```python
from build123d import *

# Parameters (mm, degrees)
EXTRUDE_1_DEPTH     = 18
SKETCH_3_W          = 20
SKETCH_3_H          = 30
EXTRUDE_2_DEPTH     = 2
SKETCH_4_W          = 4.85
SKETCH_4_H          = 30
EXTRUDE_3_DEPTH     = 6.5
EXTRUDE_START       = -20
SKETCH_5_W          = 3
SKETCH_5_H          = 12
EXTRUDE_4_DEPTH     = 20
SKETCH_2_R          = 1.25
CUT_EXTRUDE_1_DEPTH = 18


with BuildPart() as part:
    # 스케치1 → 보스-돌출1 (new body)
    with BuildSketch(Plane.XY):
        Polygon((-15, 12), (-15, 0), (15, 0), (15, 12), (11, 12), (11, 5), (-11, 5), (-11, 12), align=None)
    extrude(amount=EXTRUDE_1_DEPTH)

    # 스케치3 → 보스-돌출2 (add)
    with BuildSketch(Plane(origin=(0, 0, 0), x_dir=(-1, 0, 0), z_dir=(0, 0, -1))):
        with Locations((5, 15)):
            Rectangle(SKETCH_3_W, SKETCH_3_H)
    extrude(amount=EXTRUDE_2_DEPTH)

    # 스케치4 → 보스-돌출3 (add)
    with BuildSketch(Plane(origin=(0, 0, -2), x_dir=(-1, 0, 0), z_dir=(0, 0, -1))):
        with Locations((5, 15)):
            Rectangle(SKETCH_4_W, SKETCH_4_H)
    extrude(amount=EXTRUDE_3_DEPTH)

    # 스케치5 → 보스-돌출4 (add)
    with BuildSketch(Plane.XY.offset(18).offset(EXTRUDE_START)):
        with Locations((-16.5, -1)):
            Rectangle(SKETCH_5_W, SKETCH_5_H)
        with Locations((6.5, -1)):
            Rectangle(SKETCH_5_W, SKETCH_5_H)
    extrude(amount=EXTRUDE_4_DEPTH)

    # 스케치2 → 컷-돌출1 (cut)
    with BuildSketch(Plane(origin=(0, 5, 0), x_dir=(1, 0, 0), z_dir=(0, 1, 0))):
        with Locations((-4.8, -11.5)):
            Circle(SKETCH_2_R)
        with Locations((4.8, -11.5)):
            Circle(SKETCH_2_R)
    extrude(amount=-CUT_EXTRUDE_1_DEPTH, mode=Mode.SUBTRACT)


solid = part.part
```
Check sheet for the modelled part. Datum: model origin and axes. Units: mm. A direction names the side the tool comes from. Round coordinates to 2 decimals unless told otherwise and drop trailing zeros. Loops run counter-clockwise (first coordinate to the right, second up) from the corner with the lowest first, then second, coordinate; pieces in that order, holes last. Notation, with made-up numbers: (43, -14) - (90, -14) arc R19 ccw to (90, 0) - close; hole circle Ø11 at (6, -29.5). An arc over 180 degrees is marked (long way). Write item = value, one per line. Start each with the question number.
Q1. Section check A-A (z = 11.5). Record the boundary of the cut face in (x, y), plus the area to 3 significant figures.
Q2. Section check B-B (x = -4.8). Record the boundary of the cut face in (y, z), plus the area to 4 significant figures.
Q3. Thickness scan on L1, parallel to X at y = -1, z = -1.5; L2, parallel to X at y = 0.5, z = 11.5; L3, parallel to X at y = 10.5, z = 14. Record the ranges inside material, lowest first.
Q4. Section check D-D (x = 0.5). Record the boundary of the cut face in (y, z).
Q5. Release check for a two-part mould opening along X. For faces 4 (the face through (5.955, 0.417, 11.979)), 5 (the face through (-18, -1, 8)), 6 (the face through (5, 17, -1)) record: pulls with the +X half, pulls with the -X half, needs draft (parallel to the pull), parting line crosses it, or undercut.
Q6. Section check C-C (y = -5). Record the boundary of the cut face in (x, z), plus the area to 3 significant figures.
Q7. Access from +Z, -Z, +X, -X, +Y, -Y to the whole of each face (thin tool, end or side, straight path). Record for faces 1 (the face through (-11, 8, 9)), 2 (the face through (12, 5, 0)), 3 (the face through (11, 9, 9)).
Q8. Depth check by flat-ended pin: P1, Ø3.5, axis at x = -16.5, z = 8, coming from the +Y side; P2, Ø1, axis at x = 5, y = -2.5, coming from the -Z side; P3, Ø0.6, axis at y = 17, z = -0.5, coming from the +X side. Enter the tip coordinate at first touch or a pass-through.
Derived:
q1.outline = (-18, -7) - (-15, -7) - (-15, 0) - (-6.05, 0) - (-6.05, 5) - (-11, 5) - (-11, 12) - (-15, 12) - (-15, 5) - (-18, 5) - close; (-3.55, 0) - (3.55, 0) - (3.55, 5) - (-3.55, 5) - close; (6.05, -7) - (8, -7) - (8, 0) - (15, 0) - (15, 12) - (11, 12) - (11, 5) - (6.05, 5) - close
q1.area = 231 mm^2
q2.outline = (0, -8.5) - (30, -8.5) - (30, 0) - (5, 0) - (5, 10.25) - (0, 10.25) - close; (0, 12.75) - (5, 12.75) - (5, 18) - (0, 18) - close
q2.area = 332.5 mm^2
q3.L1 = -18 to -15, 5 to 8
q3.L2 = -18 to -6.05, -3.55 to 3.55, 6.05 to 15
q3.L3 = -15 to -11, 11 to 15
q4.outline = (0, -2) - (30, -2) - (30, 0) - (5, 0) - (5, 18) - (0, 18) - close
q5.face_4 = undercut
q5.face_5 = pulls with the -X half
q5.face_6 = pulls with the +X half
q6.outline = (-18, -2) - (-15, -2) - (-15, 18) - (-18, 18) - close; (5, -2) - (8, -2) - (8, 18) - (5, 18) - (5, 12.73) arc R1.25 cw to (5, 10.27) - close
q6.area = 118 mm^2
q7.face_1 = +Z, +Y
q7.face_2 = -Z, +X, +Y, -Y
q7.face_3 = +Z, -Z, +Y
q8.P1 = 12
q8.P2 = -2
q8.P3 = 5
